Here's how the part is built. I have some questions about the finished solid (model axes, mm). A direction names the side the tool comes from. Give positions to 0.01 mm unless a question says otherwise; leave off trailing zeros. Write each loop counter-clockwise with the first axis right and the second up, starting at its lowest first coordinate (ties: lowest second). Pieces come first, ordered by that corner, then holes. Notation, with made-up numbers: (0, 65) -> (27, 65) arc R24 cw to (27, 99) -> close; hole circle Ø5 at (79, 32.25). An arc over 180 degrees is marked (long way). Return JSON: item names as keys, results as strings.
from build123d import *
from build123d import SkipClean  # not in build123d's __all__

# Parameters (mm, degrees)
F0_W        = 15
F0_H        = 4
F1_DEPTH    = 10
F2_T4_DEPTH = 20
F3_R        = 1.5
F4_DEPTH    = 4
F5_DEPTH    = 4
F7_DEPTH    = 20
F8_W        = 56
F8_H        = 12
F9_DEPTH    = 30
F10_R       = 1.5
F11_DEPTH   = 26


# Not quite as in the source:
# - a fillet or chamfer that OpenCascade refuses, or shapes differently, is made with other operations: its cross-section is extruded or revolved along the edge and cut away or added


with BuildPart() as f1:
    # F0 (on Front) → F1 (new body, symmetric)
    with BuildSketch(Plane.XZ):
        Polygon((-74.4146332145, 2), (-74.4146332145, 0), (5.5853667855, 0), (5.5853667855, 4), (-70.4146332145, 4), (-70.4146332145, 30), (-74.4146332145, 30), (-74.4146332145, 28), (-74.4146332145, 24), (-74.4146332145, 6), align=None)
        with Locations((-81.9146332145, 26)):
            Rectangle(F0_W, F0_H)
        with Locations((-81.9146332145, 4)):
            Rectangle(F0_W, F0_H)
    extrude(amount=F1_DEPTH, both=True)

    # F2: chamfer of 30 x 60 on 1 edges, made by hand


with BuildPart() as f2_tool2:
    # F2_s3 → F2_t4 (new body)
    with BuildSketch(Plane.XZ.offset(10)):
        Polygon((-70.4146332145, 34), (-10.4146332145, 4), (-70.4146332145, 4), align=None)
    extrude(amount=-F2_T4_DEPTH)

    split(bisect_by=Plane.XY.offset(30), keep=Keep.BOTTOM)


with BuildPart() as f1_1:
    add(f1.part, clean=False)

    # F2_t1: union F2_tool2
    add(f2_tool2.part)

    # F3 (on face) → F4 (join)
    with BuildSketch(Plane.XY.offset(4)):
        with BuildLine():
            ThreePointArc((-6.1019262586, -10), (8.7805353157, -12.6258718383), (17.0853667855, 0))
            ThreePointArc((17.0853667855, 0), (8.7805353157, 12.6258718383), (-6.1019262586, 10))
            Line((-6.1019262586, 10), (1.9211532232, 10))
            ThreePointArc((1.9211532232, 10), (3.3353667855, 11), (4.7495803479, 10))
            Line((4.7495803479, 10), (5.5853667855, 10))
            Line((5.5853667855, 10), (5.5853667855, -10))
            Line((5.5853667855, -10), (4.7495803479, -10))
            ThreePointArc((4.7495803479, -10), (3.3353667855, -11), (1.9211532232, -10))
            Line((1.9211532232, -10), (-6.1019262586, -10))
        make_face()
        with Locations((11.3353667855, 0)):
            Circle(F3_R, mode=Mode.SUBTRACT)
    extrude(amount=-F4_DEPTH)

    # F3 (on face) → F5 (cut)
    with BuildSketch(Plane.XY.offset(4)):
        with Locations((-4.6646332145, 0)):
            Circle(F3_R)
        with BuildLine():
            ThreePointArc((4.8353667855, -9.5), (3.0817138174, -8.0216021605), (1.9211532232, -10))
            Line((1.9211532232, -10), (4.7495803479, -10))
            ThreePointArc((4.7495803479, -10), (4.813764625, -9.7536529681), (4.8353667855, -9.5))
        make_face()
        with BuildLine():
            Line((4.7495803479, 10), (1.9211532232, 10))
            ThreePointArc((1.9211532232, 10), (3.0817138174, 8.0216021605), (4.8353667855, 9.5))
            ThreePointArc((4.8353667855, 9.5), (4.813764625, 9.7536529681), (4.7495803479, 10))
        make_face()
    with SkipClean():  # cleaning this boolean's faces spoils the solid; the shape is the same uncleaned
        extrude(amount=-F5_DEPTH, mode=Mode.SUBTRACT)

    # F6 (on face) → F7 (cut)
    with BuildSketch(Plane.XZ.offset(10)):
        Polygon((-27.3589051245, 8), (-66.4146332145, 26), (-66.4146332145, 8), align=None)
    extrude(amount=-F7_DEPTH, mode=Mode.SUBTRACT)

    # F8 (on face) → F9 (cut)
    with BuildSketch(Plane(origin=(0, 0, 0), x_dir=(1, 0, 0), z_dir=(0, 0, -1))):
        with Locations((-42.4146332145, 0)):
            Rectangle(F8_W, F8_H)
    extrude(amount=-F9_DEPTH, mode=Mode.SUBTRACT)

    # F10 (on face) → F11 (cut)
    with BuildSketch(Plane.XY.offset(28)):
        with Locations((-84.4146332145, 5)):
            Circle(F10_R)
        with Locations((-84.4146332145, -5)):
            Circle(F10_R)
        with Locations((-79.4146332145, 0)):
            Circle(F10_R)
    extrude(amount=-F11_DEPTH, mode=Mode.SUBTRACT)


solid = f1_1.part
1. If we mould it in two halves opening along X, with no side actions, what happens to faces 1 (the face through (-82, 0, 24)), 2 (the face through (-74.415, 0, 29)), 3 (the face through (-49, -6, 5))? For each: released by +X, released by -X, zero draft, split by the parting line, or undercut.
Taken from the geometry:
{"face 1": "zero draft", "face 2": "released by -X", "face 3": "undercut"}
2. Suppose I cut it at C-C, the plane y = 2.5. List the corners of the cut face in (x, z) for me.
Taken from the geometry:
{"outline": "(-89.41, 2) -> (-74.41, 2) -> (-74.41, 0) -> (-70.41, 0) -> (-70.41, 30) -> (-74.41, 30) -> (-74.41, 28) -> (-89.41, 28) -> (-89.41, 24) -> (-74.41, 24) -> (-74.41, 6) -> (-89.41, 6) -> close; (-14.41, 0) -> (16.86, 0) -> (16.86, 4) -> (-10.41, 4) -> (-14.41, 6) -> close"}
3. Suppose I cut it at A-A, the plane z = 12.5. List the corners of the cut face in (x, y) for me.
Taken from the geometry:
{"outline": "(-74.41, -10) -> (-66.41, -10) -> (-66.41, -6) -> (-70.41, -6) -> (-70.41, 6) -> (-66.41, 6) -> (-66.41, 10) -> (-74.41, 10) -> close; (-37.12, -10) -> (-27.41, -10) -> (-27.41, -6) -> (-37.12, -6) -> close; (-37.12, 6) -> (-27.41, 6) -> (-27.41, 10) -> (-37.12, 10) -> close"}
4. Suppose I cut it at D-D, the plane z = 7. List the corners of the cut face in (x, y) for me.
Taken from the geometry:
{"outline": "(-74.41, -10) -> (-16.41, -10) -> (-16.41, -6) -> (-70.41, -6) -> (-70.41, 6) -> (-16.41, 6) -> (-16.41, 10) -> (-74.41, 10) -> close"}
5. Which directions (+Z, -Z, +X, -X, +Y, -Y) give clear straight access to the entire face, cutting with the end or side of a thin tool? Please do faces 4 (the face through (-49, 6, 5)), 5 (the face through (-82, 0, 2)), 6 (the face through (-46.613, -8.028, 16.874)).
Taken from the geometry:
{"face 4": "+Z, -Z", "face 5": "-Z, -X, +Y, -Y", "face 6": "+Y, -Y"}
6. If I drill on line 1 (Y direction, x = -32, z = 1.5); line 2 (Z direction, x = -82, y = -4.25); line 3 (X direction, y = 3, z = 11.25), over which ranges is the centre line in solid material (lowest first)? Write a range as [from, to].
Taken from the geometry:
{"line 1": "y = [-10, -6], [6, 10]", "line 2": "z = [2, 6], [24, 28]", "line 3": "x = [-74.41, -70.41]"}
7. For pin 1 Ø2 at (x, y) = (-55, -9) entering from +Z; pin 2 Ø6 at (y, z) = (-4.5, 22) entering from -X; pin 3 Ø6 at (x, z) = (-15.5, 11) entering from -Y; pin 4 Ø3 at (y, z) = (-4, 21.5) entering from +X, each with a flat end and sliding along its axis, tell me the tip position at first contact or that it passes through.
Taken from the geometry:
{"pin 1": "stops at z = 26.79", "pin 2": "stops at x = -89.41", "pin 3": "passes through", "pin 4": "stops at x = -70.41"}
8. Suppose I cut it at B-B, the plane x = -29. List the corners of the cut face in (y, z) for me, and give its area (3 significant figures).
Taken from the geometry:
{"outline": "(-10, 0) -> (-6, 0) -> (-6, 8) -> (-10, 8) -> close; (-10, 8.76) -> (-6, 8.76) -> (-6, 13.29) -> (-10, 13.29) -> close; (6, 0) -> (10, 0) -> (10, 8) -> (6, 8) -> close; (6, 8.76) -> (10, 8.76) -> (10, 13.29) -> (6, 13.29) -> close", "area": "100 mm²"}
